Geometry check sheet. Reference: the model listing, model coordinates, mm. Coordinates: 2 decimals unless noted, no trailing zeros. Loops run counter-clockwise (first coordinate to the right, second up) from the corner with the lowest first, then second, coordinate; pieces in that order, holes last. Notation, with made-up numbers: (-4, -3) - (24, -3) arc R15 cw to (24, 1) - close; hole circle Ø10 at (3, 40.25). An arc over 180 degrees is marked (long way). Write item = value, one per line. Start each with the question number.
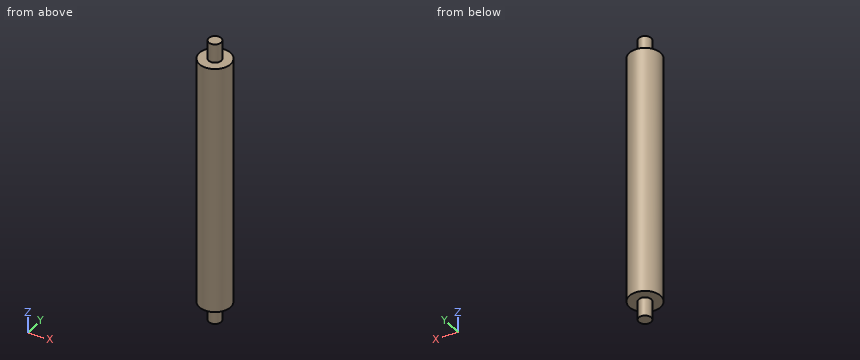
Autodesk Inventor part; units mm, degrees
ref_plane "YZ Plane" through (0, 0, 0) normal (1, 0, 0) x (0, 1, 0)
ref_plane "XZ Plane" through (0, 0, 0) normal (0, 1, 0) x (-1, 0, 0)
ref_plane "XY Plane" through (0, 0, 0) normal (0, 0, 1) x (1, 0, 0)
sketch "Sketch1" plane through (0, 0, 0) normal (0, 0, 1) x (1, 0, 0)
  circle A0 centre (0, 0) radius 2.5
  dimension "d0" = 5
extrude "Extrusion1" add sketch "Sketch1" along normal blind 40
sketch "Sketch2" plane through (0, 0, 40) normal (0, 0, 1) x (1, 0, 0)
  circle A0 centre (0, 0) radius 2.5
  circle A1 centre (0, 0) radius 1
  dimension "d3" = 2
extrude "Extrusion2" add sketch "Sketch2" along normal blind 3 contours A1
sketch "Sketch3" plane through (0, 0, 0) normal (0, 0, -1) x (-1, 0, 0)
  circle A0 centre (0, 0) radius 1
  dimension "d6" = 2
extrude "Extrusion3" add sketch "Sketch3" along normal blind 3
properties part number "Bone-4cm"
(1) Sectioned sample at A-A on x = 0. Enter the section's corners in (y, z), plus the area to 3 significant figures.
(2) Sectioned sample at C-C on z = 13. Enter the section's corners in (x, y), plus the area to 3 significant figures.
(3) Scan lines: line 1 (Z direction, x = -0.8, y = -1.4); line 2 (Y direction, x = 1.65, z = 15); line 3 (Y direction, x = -1.25, z = 13.5). Record each from-to range of solid material in increasing order.
(4) Depth check by flat-ended pin: pin 1 (2 mm diameter, centred on x = -1.5, y = 0, fed in from -Z). Enter the tip coordinate at first touch or a pass-through.
Working result:
q1.outline = (-2.5, 0) - (-1, 0) - (-1, -3) - (1, -3) - (1, 0) - (2.5, 0) - (2.5, 40) - (1, 40) - (1, 43) - (-1, 43) - (-1, 40) - (-2.5, 40) - close
q1.area = 212 mm2
q2.outline = circle Ø5 at (0, 0)
q2.area = 19.6 mm2
q3.line_1 = 0 to 40
q3.line_2 = -1.88 to 1.88
q3.line_3 = -2.17 to 2.17
q4.pin_1 = -3
